The model under review builds one solid part; all positions refer to its coordinate system, in mm. A direction names the side the tool comes from. Round coordinates to 2 decimals unless told otherwise and drop trailing zeros. Order: outer loops, then holes, each group sorted by start corner. A loop starts at its lowest first (then second) coordinate and runs counter-clockwise, first axis right, second up.
1) Mouldability with a two-part tool opening along X and no side actions: class faces 4 (the face through (0, 0, 73)), 5 (the face through (0, 0, 9)), 6 (the face through (1.5, 0, 75)), 7 (the face through (2, 0, 80)) as pulls with the +X half, pulls with the -X half, needs draft (parallel to the pull), parting line crosses it, or undercut.
2) To check wall thickness, follow L1, parallel to Z at x = -2.95, y = 0; L2, parallel to Z at x = -2.15, y = 0; L3, parallel to Z at x = 2.5, y = 0. State the ranges of each line that lie inside material, in increasing order.
3) Consider section A-A (y = 0). Give the boundary of the cut face in (x, z), then the cut area to 3 significant figures.
4) Consider section B-B (z = 5). Give the boundary of the cut face in (x, y), then the cut area to 3 significant figures.
5) Consider section C-C (x = -1.75). Give the boundary of the cut face in (y, z).
6) Clearance check with flat-ended pins moving along their axes: P1, Ø3, axis at y = -0.5, z = 77, coming from the +X side; P2, Ø2, axis at y = 0, z = 77.5, coming from the +X side; P3, Ø1.2, axis at x = 0.5, y = 0, coming from the +Z side; P4, Ø1.5, axis at x = 1, z = 35.5, coming from the +Y side. State where each tip first meets the part, or that it passes through.
7) Consider section D-D (z = 13.5). Give the boundary of the cut face in (x, y).
8) Machinability: for faces 1 (the face through (2, 0, 18)), 2 (the face through (2.486, -0.601, 75.592)), 3 (the face through (-2.5, 0, 76)), which of the approach directions +Z, -Z, +X, -X, +Y, -Y give a long, thin tool a straight path to every point of the face, cutting with its end or side? Answer none if there is none.
Autodesk Inventor part; units mm, degrees
ref_plane "YZ Plane" through (0, 0, 0) normal (1, 0, 0) x (0, 1, 0)
ref_plane "XZ Plane" through (0, 0, 0) normal (0, 1, 0) x (-1, 0, 0)
ref_plane "XY Plane" through (0, 0, 0) normal (0, 0, 1) x (1, 0, 0)
sketch "Sketch1" plane through (0, 0, 0) normal (0, 0, 1) x (1, 0, 0)
  circle A0 centre (0, 0) radius 4
  dimension "d0" = 8
extrude "Extrusion1" add sketch "Sketch1" along normal blind 80
sketch "Sketch2" plane through (0, 0, 0) normal (0, 1, 0) x (-1, 0, 0)
  line L0 (0, 0) -> (-5.3393, 0)
  line L1 (-5.3393, 0) -> (-5.3393, 18)
  line L2 (-5.3393, 18) -> (0, 18)
  line L3 (0, 18) -> (0, 0)
  line L4 (2.5, 80) -> (-1.5, 80)
  line L5 (-1.5, 80) -> (-1.5, 73)
  line L6 (-1.5, 73) -> (2.5, 73)
  line L7 (2.5, 73) -> (2.5, 80)
  line L8 (4, 80) -> (-4, 80) construction
  line L9 (-4, 80) -> (-3.5, 80)
  line L10 (-3.5, 80) -> (-3.5, 73)
  line L11 (-3.5, 73) -> (-4, 73)
  line L12 (-4, 73) -> (-4, 80)
  point P0 (-3.75, 73)
  dimension "d3" = 4
  dimension "d4" = 7
  dimension "d5" = 2.5
  dimension "d6" = 18
  dimension "d9" = 2
extrude "Extrusion2" cut sketch "Sketch2" along normal through all both and the other way through all
sketch "Sketch3" plane through (3.5, -1.9365, 73) normal (1, 0, 0) x (0, 0, -1)
  circle A0 centre (-4.5, 1.9365) radius 1.5
  line L0 (-7, 0) -> (-7, 3.873)
  point P0 (73, 1.9365)
  point P1 (-7, 1.9365)
  dimension "d10" = 3
  dimension "d11" = 2.5
hole "Hole1" at (3.5, 0, 77.5) direction (-1, 0, 0) diameter 2.459 end through all counterbore diameter 4 counterbore depth 3
sketch "Sketch4" plane through (0, -4, 18) normal (1, 0, 0) x (0, 0, -1)
  circle A0 centre (13, 4) radius 2.5
  line L0 (18, 8) -> (18, 0)
  point P0 (18, 4)
  dimension "d19" = 5
  dimension "d22" = 5
extrude "Extrusion3" cut sketch "Sketch4" against normal through all
properties part number "Servo_Strut" material "Steel, Carbon"
Answer below:
1. face 4: undercut
1. face 5: pulls with the +X half
1. face 6: undercut
1. face 7: needs draft
2. L1: z = 0 to 2.5, 7.5 to 76.27, 78.73 to 80
2. L2: z = 0 to 2.5, 7.5 to 73
2. L3: z = 18 to 75.5, 79.5 to 80
3. outline: (-4, 0) - (0, 0) - (0, 2.5) - (-4, 2.5) - close; (-4, 7.5) - (0, 7.5) - (0, 18) - (4, 18) - (4, 73) - (3.5, 73) - (3.5, 75.5) - (1.5, 75.5) - (1.5, 73) - (-2.5, 73) - (-2.5, 76.27) - (-4, 76.27) - close; (-4, 78.73) - (-2.5, 78.73) - (-2.5, 80) - (-4, 80) - close; (1.5, 79.5) - (3.5, 79.5) - (3.5, 80) - (1.5, 80) - close
3. area: 505 mm2
4. outline: (-3.12, -2.5) arc R4 ccw to (0, -4) - (0, -2.5) - close; (-3.12, 2.5) - (0, 2.5) - (0, 4) arc R4 ccw to start
4. area: 6.52 mm2
5. outline: (-3.6, 0) - (3.6, 0) - (3.6, 73) - (-3.6, 73) - close; hole circle Ø5 at (0, 5)
6. P1: stops at x = 3.5
6. P2: passes through
6. P3: stops at z = 73
6. P4: stops at y = 3.99
7. outline: (0, -4) - (0, 4) arc R4 ccw to start
8. face 1: -Z, +X, +Y, -Y
8. face 2: +X
8. face 3: +Z, +Y, -Y
